Here's how the part is built. I have some questions about the finished solid (model axes, mm). Face numbers are marked on the shaded views. A direction names the side the tool comes from. Round coordinates to 2 decimals unless told otherwise and drop trailing zeros. Order: outer loops, then holes, each group sorted by start corner. A loop starts at its lowest first (then second) coordinate and runs counter-clockwise, first axis right, second up. Notation, with made-up numbers: M 6.25,38.5 L 10.25,38.5 A21 ccw 10.25,73.5 Z; hole C 47,70.5 d5. An arc over 180 degrees is marked long. Answer as CSV lines item,"result". Start each with the question number.
```python
from build123d import *

# Parameters (mm, degrees)
EXTRUDE_1_DEPTH     = 10
CHAMFER_1_SIZE      = 2
CUT_EXTRUDE_1_DEPTH = 5


with BuildPart() as part:
    # 草图1 → 凸台-拉伸1 (new body)
    with BuildSketch(Plane(origin=(0, 0, 0), x_dir=(1, 0, 0), z_dir=(0, 1, 0))):
        with BuildLine():
            Line((0, 6), (20, 6))
            ThreePointArc((20, 6), (26, 0), (20, -6))
            Line((20, -6), (0, -6))
            ThreePointArc((0, -6), (-6, 0), (0, 6))
        make_face()
    extrude(amount=EXTRUDE_1_DEPTH)

    # 草图2 → 切除-旋转1 (revolve, cut)
    with BuildSketch(Plane.XY, mode=Mode.PRIVATE) as cut_revolve_1_sk:
        Polygon((-2.55, 10), (-2.55, 5), (-1.6, 5), (-1.6, 2), (-2.55, 2), (-2.55, 0), (0, 0), (0, 10), align=None)
    revolve(cut_revolve_1_sk.sketch.rotate(Axis((0, 0, 0), (0, 1, 0)), 270), axis=Axis((0, 0, 0), (0, 1, 0)), mode=Mode.SUBTRACT)

    # 草图3 → 切除-旋转2 (revolve, cut)
    with BuildSketch(Plane.XY, mode=Mode.PRIVATE) as cut_revolve_2_sk:
        Polygon((20, 0), (17.425, 0), (17.425, 5), (17, 5), (17, 10), (20, 10), align=None)
    revolve(cut_revolve_2_sk.sketch.rotate(Axis((20, 10, 0), (0, -1, 0)), 270), axis=Axis((20, 10, 0), (0, -1, 0)), mode=Mode.SUBTRACT)

    # 倒角1
    # the kernel refuses this chamfer: 2 mm, written as the material it takes off along each edge
    with BuildSketch(Plane(origin=(20, 10, 0), x_dir=(0, 0, -1), z_dir=(-1, 0, 0))) as chamfer_1_piece_1:
        Polygon((6, CHAMFER_1_SIZE), (6 - CHAMFER_1_SIZE, 0), (6, 0), align=None)
    revolve(axis=Axis((20, 10, 0), (0, -1, 0)), revolution_arc=180, mode=Mode.SUBTRACT)
    with BuildSketch(Plane(origin=(0, 10, 0), x_dir=(0, 0, -1), z_dir=(1, 0, 0))) as chamfer_1_piece_2:
        Polygon((2.55 + CHAMFER_1_SIZE, 0), (2.55, -CHAMFER_1_SIZE), (2.55, 0), align=None)
    revolve(axis=Axis((0, 10, 0), (0, 1, 0)), mode=Mode.SUBTRACT)
    with BuildSketch(Plane(origin=(0, 10, -6), x_dir=(0, -0.9996219169112968, -0.027495876610586487), z_dir=(1, 0, 0)), Plane(origin=(20, 10, 6), x_dir=(0, -0.9996219169112968, 0.027495876610586487), z_dir=(-1, 0, 0))) as chamfer_1_piece_3:
        Polygon((CHAMFER_1_SIZE * 0.999621916911, -CHAMFER_1_SIZE * 0.0274958766106), (-CHAMFER_1_SIZE * 0.0274958766106, -CHAMFER_1_SIZE * 0.999621916911), (0, 0), align=None)
    extrude(amount=20, mode=Mode.SUBTRACT)
    with BuildSketch(Plane(origin=(20, 10, 0), x_dir=(0, 0, 1), z_dir=(1, 0, 0))) as chamfer_1_piece_4:
        Polygon((3 + CHAMFER_1_SIZE, 0), (3, CHAMFER_1_SIZE), (3, 0), align=None)
    revolve(axis=Axis((20, 10, 0), (0, -1, 0)), mode=Mode.SUBTRACT)
    with BuildSketch(Plane(origin=(0, 10, 0), x_dir=(0, 0, 1), z_dir=(1, 0, 0))) as chamfer_1_piece_5:
        Polygon((6 - CHAMFER_1_SIZE, 0), (6, CHAMFER_1_SIZE), (6, 0), align=None)
    revolve(axis=Axis((0, 10, 0), (0, -1, 0)), revolution_arc=180, mode=Mode.SUBTRACT)

    # 草图4 → 切除-拉伸1 (cut)
    with BuildSketch(Plane.XZ):
        Polygon((-2.107328483, -3.65), (2.107328483, -3.65), (4.214656965, 0), (2.107328483, 3.65), (-2.107328483, 3.65), (-4.214656965, 0), align=None)
    extrude(amount=-CUT_EXTRUDE_1_DEPTH, mode=Mode.SUBTRACT)


solid = part.part
```
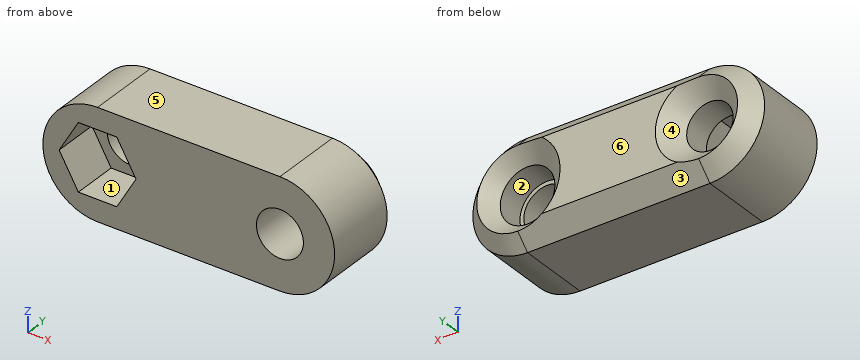
Item 1: If we section it at B-B on x = 9: Please give me the cut outline in (y, z).
Item 2: We'd pull the mould along Z, two halves only. Please class the marked faces 4, 5 and 6: pulls with the +Z half, pulls with the -Z half, needs draft (parallel to the pull), parting line crosses it, or undercut.
Item 3: If I drill on line 1 along X through (y, z) = (7.3, 0); line 2 along X through (y, z) = (1.25, 1); line 3 along Z through (x, y) = (20, 3.6) (3 decimals), over which ranges is the centre line in solid material (lowest first)?
Item 4: If we section it at C-C on y = 8.5: Please give me the cut outline in (x, z).
Item 5: If we section it at D-D on z = 1.5: Count the separate pieces of the cut face and the enclosed holes in it, and give its area (3 significant figures).
Item 6: For P1, Ø2, axis at x = -0.5, z = 1.5, coming from the -Y side; P2, Ø2, axis at y = 1.5, z = -4, coming from the -X side, each with a flat end and sliding along its axis, tell me the tip position at first contact or that it passes through.
Item 7: If we section it at A-A on y = 3: Please give me the cut outline in (x, z) (3 decimals).
Item 8: Which directions (+Z, -Z, +X, -X, +Y, -Y) give clear straight access to the entire face, cutting with the end or side of a thin tool? Please do the marked faces 1, 2 and 3.
Geometry says:
1,outline,"M 0,-6 L 8,-6 L 10,-4 L 10,4 L 8,6 L 0,6 Z"
2,face 4,"undercut"
2,face 5,"pulls with the +Z half"
2,face 6,"needs draft"
3,line 1,"-6 to -2.55, 2.55 to 17, 23 to 26"
3,line 2,"-5.92 to -3.64, 3.64 to 17.63, 22.37 to 25.92"
3,line 3,"-6 to -2.575, 2.575 to 6"
4,outline,"M 0,-5.5 L 20,-5.5 A5.5 ccw 20,5.5 L 0,5.5 A5.5 ccw Z; hole C 0,0 d6.1; hole C 20,0 d7"
5,separate pieces,"3"
5,enclosed holes,"0"
5,area,"202 mm²"
6,P1,"y = 5"
6,P2,"x = -5.2"
7,outline,"M 0,-6 L 20,-6 A6 ccw 20,6 L 0,6 A6 ccw Z; hole M -4.215,0 L -2.107,-3.65 L 2.107,-3.65 L 4.215,0 L 2.107,3.65 L -2.107,3.65 Z; hole C 20,0 d5.15"
8,face 1,"-Y"
8,face 2,"+Y"
8,face 3,"-Z, +X, -X, +Y"
